Study the drawing (mm; zero at the part's minimum x, y, z) and answer. A direction names the side the tool comes from. Round coordinates to 2 decimals unless told otherwise and drop trailing zeros. Write each loop counter-clockwise with the first axis right and the second up, starting at its lowest first coordinate (ties: lowest second). Pieces come first, ordered by that corner, then holes. Notation, with made-up numbers: (67, -10.75) - (119, -10.75) arc R25 ccw to (119, 27.25) - close; hole circle Ø9 at (-6, -40). An arc over 180 degrees is marked (long way). Use one line per item in the form item = value. Start each with the question number.
1) The part is cut by section C-C, the plane y = 44. Give the vertices of the cut face in (x, z).
2) For the marked faces 1 and 2, determine the directions among +Z, -Z, +X, -X, +Y, -Y from which every point of the face is accessible in a straight line to the end or side of a thin tool.
3) Consider line 1 along X through (y, z) = (43.5, 64); line 2 along Z through (x, y) = (46, 20.5); line 3 along X through (y, z) = (43.5, 5.5). Determine where each line is inside the solid, lowest interval first. Write a range as from..to.
4) The part is cut by section A-A, the plane x = 26. Give the vertices of the cut face in (y, z), plus the area to 4 significant figures.
5) The part is cut by section B-B, the plane y = 32.75. Give the vertices of the cut face in (x, z), plus the area to 3 significant figures.
6) The part is cut by section D-D, the plane x = 13.5. Give the vertices of the cut face in (y, z).
7) Each of these flat-tipped pins is pushed along its axis until it touches: pin 1 (4 mm diameter, centred on y = 50.5, z = 20, fed in from +X); pin 2 (10 mm diameter, centred on x = 20, y = 34.5, fed in from +Z). Where does it stop, or does it pass through?
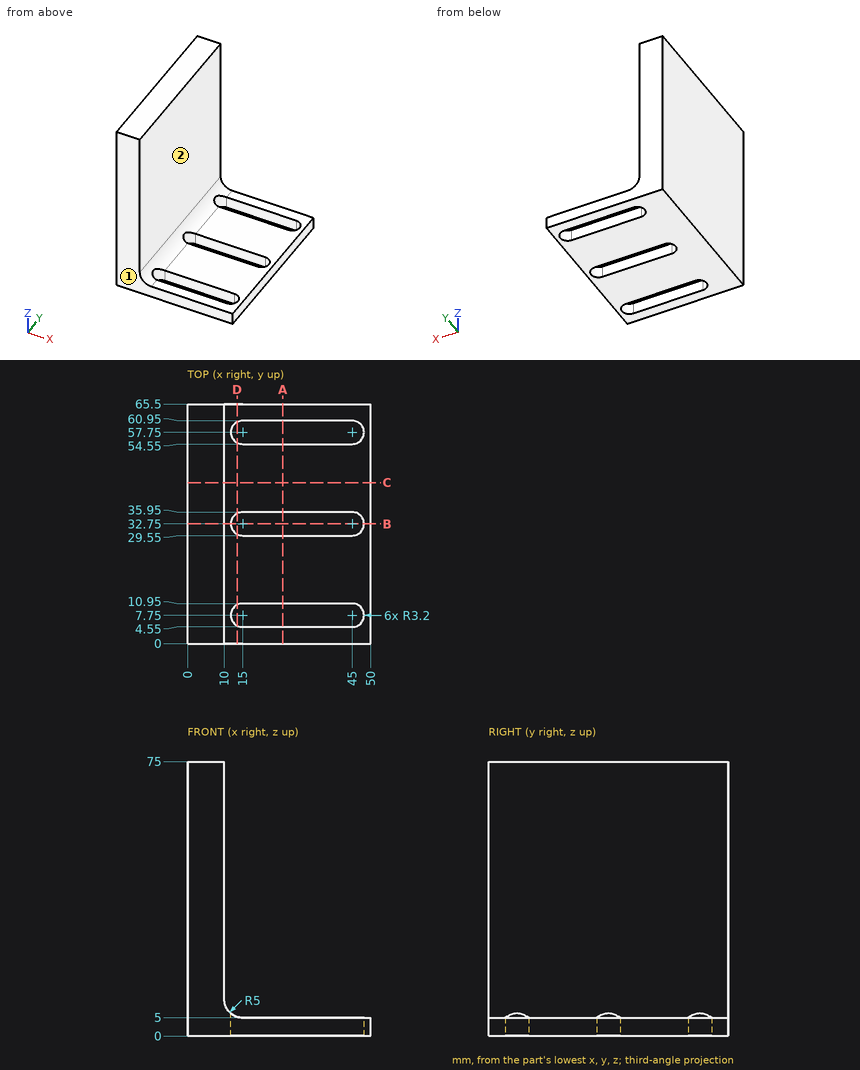
Geometry results:
q1.outline = (0, 0) - (50, 0) - (50, 5) - (15, 5) arc R5 cw to (10, 10) - (10, 75) - (0, 75) - close
q2.face_1 = +Z, -Z, +X, -X, -Y
q2.face_2 = +Z, +X, +Y, -Y
q3.line_1 = 0..10
q3.line_2 = 0..5
q3.line_3 = 0..12.82
q4.outline = (0, 0) - (4.55, 0) - (4.55, 5) - (0, 5) - close; (10.95, 0) - (29.55, 0) - (29.55, 5) - (10.95, 5) - close; (35.95, 0) - (54.55, 0) - (54.55, 5) - (35.95, 5) - close; (60.95, 0) - (65.5, 0) - (65.5, 5) - (60.95, 5) - close
q4.area = 231.5 mm2
q5.outline = (0, 0) - (11.8, 0) - (11.8, 6.16) arc R5 cw to (10, 10) - (10, 75) - (0, 75) - close; (48.2, 0) - (50, 0) - (50, 5) - (48.2, 5) - close
q5.area = 772 mm2
q6.outline = (0, 0) - (4.92, 0) - (4.92, 5.23) - (0, 5.23) - close; (10.58, 0) - (29.92, 0) - (29.92, 5.23) - (10.58, 5.23) - close; (35.58, 0) - (54.92, 0) - (54.92, 5.23) - (35.58, 5.23) - close; (60.58, 0) - (65.5, 0) - (65.5, 5.23) - (60.58, 5.23) - close
q7.pin_1 = 10
q7.pin_2 = 5
